The figure shows three views and two pictorial views of one solid part (mm, origin at its lowest corner). Answer the questions. A direction names the side the tool comes from. Give positions to 0.01 mm unless a question says otherwise; leave off trailing zeros. Write each loop counter-clockwise with the first axis right and the second up, starting at its lowest first coordinate (ties: lowest second). Pieces come first, ordered by that corner, then holes. Notation, with made-up numbers: (7.25, 64) - (11.25, 64) arc R12 ccw to (11.25, 70) - close; hole circle Ø1 at (35, 55.25). An arc over 180 degrees is marked (long way). Write each question's results on one line, items separated by ' | '. Start each with the question number.
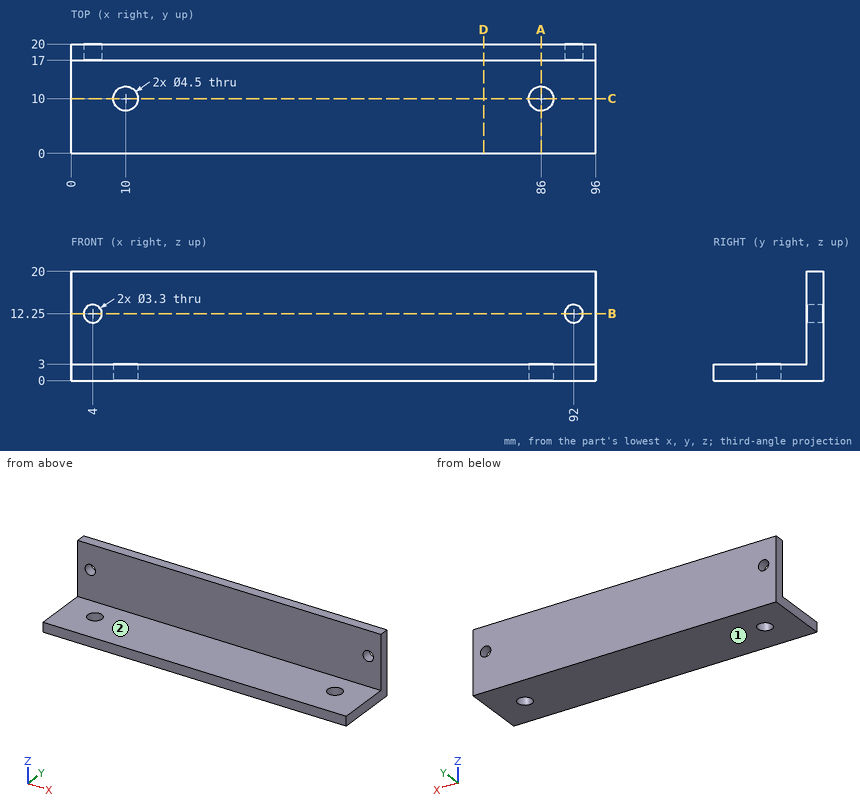
Q1. A cutting plane is placed at A-A, the plane x = 86. Write down the section's boundary in (y, z).
Q2. A cutting plane is placed at B-B, the plane z = 12.25. Write down the section's boundary in (x, y).
Q3. A tool of negligible diameter and unlimited length cuts with its end or side. For the marked faces 1 and 2, from which of +Z, -Z, +X, -X, +Y, -Y can it reach the whole face along a straight path? Write none if from no direction.
Q4. A cutting plane is placed at C-C, the plane y = 10. Write down the section's boundary in (x, z).
Q5. Consider L1, parallel to X at y = 18.45, z = 12.25; L2, parallel to Z at x = 4, y = 17.7; L3, parallel to Y at x = 10, z = 0.65. Determine where each line is inside the solid, lowest interval first.
Q6. Given pin 1 (10 mm diameter, centred on y = 11, z = 7.5, fed in from -X); pin 2 (8.5 mm diameter, centred on x = 50, z = 15, fed in from -Y); pin 3 (7 mm diameter, centred on x = 10, y = 10, fed in from +Z), each flat-ended and moving along its own axis, determine where each tip first touches the part or whether it passes through.
Q7. A cutting plane is placed at D-D, the plane x = 75.5. Write down the section's boundary in (y, z), and give its area (3 significant figures).
Result:
1) outline: (0, 0) - (7.75, 0) - (7.75, 3) - (0, 3) - close; (12.25, 0) - (20, 0) - (20, 20) - (17, 20) - (17, 3) - (12.25, 3) - close
2) outline: (0, 17) - (2.35, 17) - (2.35, 20) - (0, 20) - close; (5.65, 17) - (90.35, 17) - (90.35, 20) - (5.65, 20) - close; (93.65, 17) - (96, 17) - (96, 20) - (93.65, 20) - close
3) face 1: -Z, +X, -X, +Y, -Y | face 2: +Z, +X, -X, -Y
4) outline: (0, 0) - (7.75, 0) - (7.75, 3) - (0, 3) - close; (12.25, 0) - (83.75, 0) - (83.75, 3) - (12.25, 3) - close; (88.25, 0) - (96, 0) - (96, 3) - (88.25, 3) - close
5) L1: x = 0 to 2.35, 5.65 to 90.35, 93.65 to 96 | L2: z = 0 to 10.6, 13.9 to 20 | L3: y = 0 to 7.75, 12.25 to 20
6) pin 1: stops at x = 0 | pin 2: stops at y = 17 | pin 3: stops at z = 3
7) outline: (0, 0) - (20, 0) - (20, 20) - (17, 20) - (17, 3) - (0, 3) - close | area: 111 mm2
